from build123d import *

# Parameters (mm, degrees)
SKETCH1_W           = 140
SKETCH1_H           = 60
BOSS_EXTRUDE1_DEPTH = 3.175
SKETCH2_W           = 20
SKETCH2_H           = 3.175
SKETCH2_W_2         = 3.175
SKETCH2_H_2         = 10
CUT_EXTRUDE1_DEPTH  = 3.175


with BuildPart() as part:
    # Sketch1 → Boss-Extrude1 (new body)
    with BuildSketch(Plane.XY):
        with Locations((5.981871877, 26.825)):
            Rectangle(SKETCH1_W, SKETCH1_H)
    extrude(amount=-BOSS_EXTRUDE1_DEPTH)

    # Sketch2 → Cut-Extrude1 (cut)
    with BuildSketch(Plane.XY):
        Polygon((-60.843128123, 0), (-44.768128123, 0), (-44.768128123, -3.175), (-64.018128123, -3.175), (-64.018128123, 0), (-64.018128123, 6.475), (-60.843128123, 6.475), align=None)
        Polygon((56.731871877, 0), (72.806871877, 0), (72.806871877, 6.675), (75.981871877, 6.675), (75.981871877, 0), (75.981871877, -3.175), (56.731871877, -3.175), align=None)
        Polygon((75.981871877, 46.975), (75.981871877, 53.65), (75.981871877, 56.825), (56.731871877, 56.825), (56.731871877, 53.65), (72.806871877, 53.65), (72.806871877, 46.975), align=None)
        with Locations((26.231871877, 55.2375)):
            Rectangle(SKETCH2_W, SKETCH2_H)
        with Locations((-14.268128123, 55.2375)):
            Rectangle(SKETCH2_W, SKETCH2_H)
        Polygon((-64.018128123, 56.825), (-64.018128123, 53.65), (-64.018128123, 47.175), (-60.843128123, 47.175), (-60.843128123, 53.65), (-44.768128123, 53.65), (-44.768128123, 56.825), align=None)
        with Locations((74.394371877, 26.825)):
            Rectangle(SKETCH2_W_2, SKETCH2_H_2)
        with Locations((-62.430628123, 26.825)):
            Rectangle(SKETCH2_W_2, SKETCH2_H_2)
        with Locations((-14.268128123, -1.5875)):
            Rectangle(SKETCH2_W, SKETCH2_H)
        with Locations((26.231871877, -1.5875)):
            Rectangle(SKETCH2_W, SKETCH2_H)
    extrude(amount=-CUT_EXTRUDE1_DEPTH, mode=Mode.SUBTRACT)


solid = part.part
Model file for the job. Use its own axes, mm. A direction names the side the tool comes from. Coordinates: 2 decimals unless noted, no trailing zeros. Loops run counter-clockwise (first coordinate to the right, second up) from the corner with the lowest first, then second, coordinate; pieces in that order, holes last. Notation, with made-up numbers: (64.25, 26) -> (119.25, 26) arc R7 ccw to (119.25, 39) -> close; hole circle Ø5 at (-25.5, 23). An arc over 180 degrees is marked (long way). Use one line per item in the form item = value. Start each with the question number.
(1) Probe probe 1 along Y at (x, z) = (-5.5, -2); probe 2 along X at (y, z) = (53.5, -1.1). List the from-to ranges inside material, lowest first. Write a range as from..to.
(2) Pull direction Y, two halves, no side cores. Call faces 4 (the flat face through (-62, 6.475, -2)), 5 (the flat face through (74, 21.825, -2)), 6 (the flat face through (75.982, 14, -2)): pulls with the +Y half, pulls with the -Y half, needs draft (parallel to the pull), parting line crosses it, or undercut.
(3) Flat gauge pins, fed straight in: pin 1 (1 mm diameter, centred on x = 74.5, z = -1.5, fed in from -Y) (3 decimals); pin 2 (1.6 mm diameter, centred on x = -63, z = -2, fed in from +Y) (3 decimals); pin 3 (1.6 mm diameter, centred on y = 3.5, z = -2, fed in from +X). Where does each tip first touch, or does it go through?
(4) Cut at B-B on y = 26. Give the cut face in (x, z) (3 decimals), and give its area (3 significant figures).
(5) Cut at A-A on x = -6.5. Give the cut face in (y, z) (3 decimals), and give its area (3 significant figures).
(6) Tool access for faces 1 (the flat face through (-53, 53.65, -2)), 2 (the flat face through (-62, 31.825, -2)), 3 (the flat face through (-53, 0, -2)): list every direction of +Z, -Z, +X, -X, +Y, -Y with a clear straight run to the whole face (end or side of a thin tool).
Values:
q1.probe_1 = 0..53.65
q1.probe_2 = -60.84..72.81
q2.face_4 = pulls with the -Y half
q2.face_5 = undercut
q2.face_6 = needs draft
q3.pin_1 = 6.675
q3.pin_2 = 47.175
q3.pin_3 = 72.81
q4.outline = (-60.843, -3.175) -> (72.807, -3.175) -> (72.807, 0) -> (-60.843, 0) -> close
q4.area = 424 mm2
q5.outline = (0, -3.175) -> (53.65, -3.175) -> (53.65, 0) -> (0, 0) -> close
q5.area = 170 mm2
q6.face_1 = +Z, -Z, -X, +Y
q6.face_2 = +Z, -Z, -X
q6.face_3 = +Z, -Z, -X, -Y
